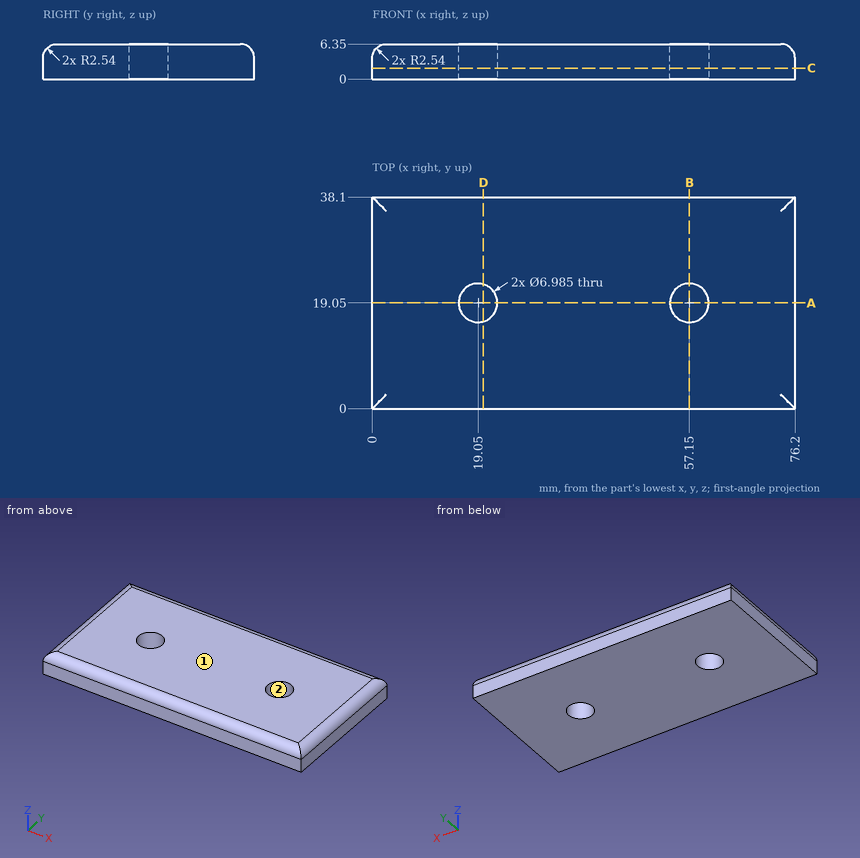
Can you work these out from the drawing? Everything is in mm from the part's minimum corner. Coordinates: 2 decimals unless noted, no trailing zeros. Loops run counter-clockwise (first coordinate to the right, second up) from the corner with the lowest first, then second, coordinate; pieces in that order, holes last.
1) Imagine slicing it at B-B on x = 57.15. List the corners of the cut face in (y, z) for me, plus the area to 3 significant figures.
2) Thinking about a two-plate mould opening in X: for the marked faces 1 and 2, which applies, pulls with the +X half, pulls with the -X half, needs draft (parallel to the pull), parting line crosses it, or undercut?
3) Imagine slicing it at C-C on z = 2. State how many separate pieces and enclosed holes the cut face has, plus the area to 3 significant figures.
4) Imagine slicing it at A-A on y = 19.05. List the corners of the cut face in (x, z) for me, plus the area to 3 significant figures.
5) Imagine slicing it at D-D on x = 20. List the corners of the cut face in (y, z) for me, plus the area to 3 significant figures.
6) I need wall thicknesses on probe 1 along X at (y, z) = (18.5, 2.75); probe 2 along Y at (x, z) = (19.05, 1.75); probe 3 along X at (y, z) = (21, 1.5). Which ranges of each line are inside material? Lowest first, please.
Completed:
1. outline: (0, 0) - (15.56, 0) - (15.56, 6.35) - (2.54, 6.35) arc R2.54 ccw to (0, 3.81) - close; (22.54, 0) - (38.1, 0) - (38.1, 3.81) arc R2.54 ccw to (35.56, 6.35) - (22.54, 6.35) - close
1. area: 195 mm2
2. face 1: needs draft
2. face 2: undercut
3. separate pieces: 1
3. enclosed holes: 2
3. area: 2,830 mm2
4. outline: (0, 0) - (15.56, 0) - (15.56, 6.35) - (2.54, 6.35) arc R2.54 ccw to (0, 3.81) - close; (22.54, 0) - (53.66, 0) - (53.66, 6.35) - (22.54, 6.35) - close; (60.64, 0) - (76.2, 0) - (76.2, 3.81) arc R2.54 ccw to (73.66, 6.35) - (60.64, 6.35) - close
4. area: 392 mm2
5. outline: (0, 0) - (15.69, 0) - (15.69, 6.35) - (2.54, 6.35) arc R2.54 ccw to (0, 3.81) - close; (22.41, 0) - (38.1, 0) - (38.1, 3.81) arc R2.54 ccw to (35.56, 6.35) - (22.41, 6.35) - close
5. area: 196 mm2
6. probe 1: x = 0 to 15.6, 22.5 to 53.7, 60.6 to 76.2
6. probe 2: y = 0 to 15.56, 22.54 to 38.1
6. probe 3: x = 0 to 16.15, 21.95 to 54.25, 60.05 to 76.2
